from build123d import *

# Parameters (mm, degrees)
SKETCH_1_W      = 412.9
SKETCH_1_H      = 81.4
SKETCH_1_R      = 2
EXTRUDE_1_DEPTH = 0.6
SKETCH_2_R      = 2
EXTRUDE_2_DEPTH = 0.6
EXTRUDE_START   = -0.6
SKETCH_3_R      = 2
EXTRUDE_3_DEPTH = 0.6


with BuildPart() as part:
    # Эскиз1 → Бобышка-Вытянуть1 (new body)
    with BuildSketch(Plane.XY):
        with Locations((241.1, 40.7)):
            Rectangle(SKETCH_1_W, SKETCH_1_H)
        with Locations((40.25, 10.7)):
            Circle(SKETCH_1_R, mode=Mode.SUBTRACT)
        with Locations((441.95, 10.7)):
            Circle(SKETCH_1_R, mode=Mode.SUBTRACT)
        with Locations((40.25, 70.7)):
            Circle(SKETCH_1_R, mode=Mode.SUBTRACT)
        with Locations((441.95, 70.7)):
            Circle(SKETCH_1_R, mode=Mode.SUBTRACT)
    extrude(amount=EXTRUDE_1_DEPTH)

    # Эскиз2 → Бобышка-Вытянуть2 (add)
    with BuildSketch(Plane(origin=(0, 81.4, 0), x_dir=(1, 0, 0), z_dir=(0, 1, 0))):
        Polygon((44.65, -0.6), (50.423502692, -10.6), (431.776497308, -10.6), (437.55, -0.6), align=None)
        with Locations(Location((401.1, -5.6, 0), (0, 0, 180))):
            Circle(SKETCH_2_R, mode=Mode.SUBTRACT)
        with Locations(Location((321.1, -5.6, 0), (0, 0, 180))):
            Circle(SKETCH_2_R, mode=Mode.SUBTRACT)
        with Locations(Location((241.1, -5.6, 0), (0, 0, 180))):
            Circle(SKETCH_2_R, mode=Mode.SUBTRACT)
        with Locations(Location((161.1, -5.6, 0), (0, 0, 180))):
            Circle(SKETCH_2_R, mode=Mode.SUBTRACT)
        with Locations(Location((81.1, -5.6, 0), (0, 0, 180))):
            Circle(SKETCH_2_R, mode=Mode.SUBTRACT)
    extrude(amount=-EXTRUDE_2_DEPTH)

    # Эскиз3 → Бобышка-Вытянуть3 (add)
    with BuildSketch(Plane.XZ.offset(EXTRUDE_START)):
        Polygon((44.65, 0.6), (437.55, 0.6), (431.776497308, 10.6), (50.423502692, 10.6), align=None)
        with Locations(Location((401.1, 5.6, 0), (0, 0, 180))):
            Circle(SKETCH_3_R, mode=Mode.SUBTRACT)
        with Locations(Location((321.1, 5.6, 0), (0, 0, 180))):
            Circle(SKETCH_3_R, mode=Mode.SUBTRACT)
        with Locations(Location((241.1, 5.6, 0), (0, 0, 180))):
            Circle(SKETCH_3_R, mode=Mode.SUBTRACT)
        with Locations(Location((161.1, 5.6, 0), (0, 0, 180))):
            Circle(SKETCH_3_R, mode=Mode.SUBTRACT)
        with Locations(Location((81.1, 5.6, 0), (0, 0, 180))):
            Circle(SKETCH_3_R, mode=Mode.SUBTRACT)
    extrude(amount=EXTRUDE_3_DEPTH)


solid = part.part
Work out the finished part from the listing and answer in its coordinate system (mm). A direction names the side the tool comes from. Coordinates: 2 decimals unless noted, no trailing zeros. Order: outer loops, then holes, each group sorted by start corner. A loop starts at its lowest first (then second) coordinate and runs counter-clockwise, first axis right, second up. Notation, with made-up numbers: (-1, 71) - (52, 71) arc R18 cw to (52, 80) - close; hole circle Ø5 at (38, 13). An arc over 180 degrees is marked (long way). Put each result on its own line as item: value. Start each with the question number.
1) Find section B-B (z = 5.6). State how many separate pieces and enclosed holes the cut face has, plus the area to 3 significant figures.
2) Find section A-A (x = 128.5). Give the vertices of the cut face in (y, z).
3) Find the intervals of material crossed by line 1 (Y direction, x = 441.95, z = 0.35); line 2 (Z direction, x = 321, y = 81); line 3 (Y direction, x = 210, z = 8.25), in increasing order. Write a range as from..to.
4) Flat-ended cylindrical pins translate along their axes: pin 1 (5 mm diameter, centred on x = 441.95, y = 70.7, fed in from +Z); pin 2 (3.5 mm diameter, centred on x = 321.1, z = 5.6, fed in from -Y). Find the tip coordinate at first contact, or state that the pin passes through.
5) Find section C-C (y = 54). Give the vertices of the cut face in (x, z), plus the area to 3 significant figures.
6) For a pull along Y with two mould halves and no side action, classify faces 1 (the flat face through (238, 41, 0)), 2 (the flat face through (238, 41, 0.6)), 3 (the flat face through (238, 81.4, 5)) as released by +Y, released by -Y, zero draft, split by the parting line, or undercut.
7) For faces 4 (the flat face through (238, 0, 5)), 5 (the flat face through (238, 0.6, 6)), determine the directions among +Z, -Z, +X, -X, +Y, -Y from which every point of the face is accessible in a straight line to the end or side of a thin tool.
Results list:
1. separate pieces: 12
1. enclosed holes: 0
1. area: 441 mm^2
2. outline: (0, 0) - (81.4, 0) - (81.4, 10.6) - (80.8, 10.6) - (80.8, 0.6) - (0.6, 0.6) - (0.6, 10.6) - (0, 10.6) - close
3. line 1: y = 0..8.7, 12.7..68.7, 72.7..81.4
3. line 2: z = 0..3.6, 7.6..10.6
3. line 3: y = 0..0.6, 80.8..81.4
4. pin 1: stops at z = 0.6
4. pin 2: passes through
5. outline: (34.65, 0) - (447.55, 0) - (447.55, 0.6) - (34.65, 0.6) - close
5. area: 248 mm^2
6. face 1: zero draft
6. face 2: undercut
6. face 3: released by +Y
7. face 4: +Z, -Z, +X, -X, -Y
7. face 5: +Z, +X, -X
